Work out the finished part from the listing and answer in its coordinate system (mm). A direction names the side the tool comes from. Coordinates: 2 decimals unless noted, no trailing zeros. Write each loop counter-clockwise with the first axis right and the second up, starting at its lowest first coordinate (ties: lowest second). Pieces come first, ordered by that corner, then holes. Notation, with made-up numbers: M 73,9 L 129,9 A22 cw 129,19 Z; hole C -30,65 d1. An arc over 180 degrees is marked long. Answer as CSV lines item,"result". Start each with the question number.
(1) A cutting plane is placed at C-C on y = 19. Give the vertices of the cut face in (x, z), then the cut area to 3 significant figures.
(2) The mould has two halves that part along Y. Classify faces 4 (the cylindrical face through (33.538, 17.004, 6.014)), 5 (the flat face through (-17.75, 22, 6)), 6 (the cylindrical face through (-19.14, -26.1, 4.04)), 7 (the conical face through (30.577, -30.812, 0.125)): released by +Y, released by -Y, zero draft, split by the parting line, or undercut.
(3) Flat-ended cylindrical pins translate along their axes: P1, Ø4, axis at x = 30, y = 17.5, coming from the +Z side; P2, Ø5, axis at x = 24, z = 7, coming from the -Y side; P3, Ø1, axis at x = -24.5, z = 7.5, coming from the -Y side. Find the tip coordinate at first contact, or state that the pin passes through.
(4) Find the intervals of material crossed by L1, parallel to Y at x = 16, z = 6.45; L2, parallel to Y at x = -11.5, z = 5.25; L3, parallel to X at y = -24.5, z = 1.5, in increasing order. Write a range as [from, to].
(5) For faces 1 (the conical face through (29.334, -29.541, 1.347)), 2 (the flat face through (-32, -30, 6)), 3 (the flat face through (-19, 22, 4)), determine the directions among +Z, -Z, +X, -X, +Y, -Y from which every point of the face is accessible in a straight line to the end or side of a thin tool.
(6) A cutting plane is placed at B-B on y = -14. Give the vertices of the cut face in (x, z), then the cut area to 3 significant figures.
(7) A cutting plane is placed at A-A on x = 7.5. Give the vertices of the cut face in (y, z), then the cut area to 3 significant figures.
(8) A cutting plane is placed at D-D on x = 16. Give the vertices of the cut face in (y, z).
from build123d import *

# Parameters (mm, degrees)
PAD_DEPTH       = 9
POCKET_DEPTH    = 8
SKETCH002_W     = 37
SKETCH002_H     = 32
POCKET001_DEPTH = 1.001
POCKET002_DEPTH = 5
SKETCH004_W     = 45
SKETCH004_H     = 5
POCKET003_DEPTH = 74.001
SKETCH005_W     = 6.5
SKETCH005_H     = 8
PAD001_DEPTH    = 6
SKETCH006_R     = 2.25
POCKET004_DEPTH = 2
CHAMFER_SIZE    = 2
CHAMFER001_SIZE = 2
FILLET_R        = 3


with BuildPart() as part:
    # Sketch → Pad (new body)
    with BuildSketch(Plane.XY):
        with BuildLine():
            Line((-37, 23), (-37, -20))
            ThreePointArc((-37, -20), (-32.020815, -32.020815), (-20, -37))
            Line((-20, -37), (20.000003, -37))
            ThreePointArc((20.000003, -37), (32.020816, -32.020814), (37, -20))
            Line((37, -20), (37, 23))
            Line((-37, 23), (37, 23))
        make_face()
    extrude(amount=PAD_DEPTH)

    # Sketch001 (on Face8 of Pad) → Pocket (cut)
    with BuildSketch(Plane.XY.offset(9)):
        with BuildLine():
            Line((-35, 21), (-35, -20))
            ThreePointArc((-35, -20), (-30.606602, -30.606602), (-20, -35))
            Line((-20, -35), (20, -35))
            ThreePointArc((20, -35), (30.606602, -30.606602), (35, -20))
            Line((35, 21), (35, -20))
            Line((-35, 21), (35, 21))
        make_face()
    extrude(amount=-POCKET_DEPTH, mode=Mode.SUBTRACT)

    # Sketch002 (on Face15 of Pocket) → Pocket001 (cut, through all)
    with BuildSketch(Plane.XY.offset(1)):
        with Locations((3, 1)):
            Rectangle(SKETCH002_W, SKETCH002_H)
    extrude(amount=-POCKET001_DEPTH, mode=Mode.SUBTRACT)

    # Sketch003 (on Face2 of Pocket001) → Pocket002 (cut)
    with BuildSketch(Plane(origin=(0, 23, 0), x_dir=(-1, 0, 0), z_dir=(0, 1, 0))):
        Polygon((-35, 9), (35, 9), (35, 7), (24.25, 7), (24.25, 5), (23, 5), (23, 3), (19, 3), (19, 5), (17.75, 5), (17.75, 7), (-17.75, 7), (-17.75, 5), (-19, 5), (-19, 3), (-23, 3), (-23, 5), (-24.25, 5), (-24.25, 7), (-35, 7), align=None)
    extrude(amount=-POCKET002_DEPTH, mode=Mode.SUBTRACT)

    # Sketch004 → Pocket003 (cut, through all)
    with BuildSketch(Plane.YZ.offset(37)):
        with Locations((-7.5, 6.5)):
            Rectangle(SKETCH004_W, SKETCH004_H)
    extrude(amount=-POCKET003_DEPTH, mode=Mode.SUBTRACT)

    # Sketch005 (on Face43 of Pocket003) → Pad001 (join)
    with BuildSketch(Plane.XY.offset(1)):
        Polygon((-20, -19), (20, -19), (20, -27), (12, -27), (12, -21), (-12, -21), (-12, -27), (-20, -27), align=None)
        with Locations((-31.75, 18.9)):
            Rectangle(SKETCH005_W, SKETCH005_H)
        with Locations((31.75, 18.9)):
            Rectangle(SKETCH005_W, SKETCH005_H)
    extrude(amount=PAD001_DEPTH)

    # Sketch006 (on Face69 of Pad001) → Pocket004 (cut)
    with BuildSketch(Plane.XY.offset(7)):
        with Locations((-16, -23)):
            Circle(SKETCH006_R)
        with Locations((16, -23)):
            Circle(SKETCH006_R)
        with Locations((-32.5, 19)):
            Circle(SKETCH006_R)
        with Locations((32.5, 19)):
            Circle(SKETCH006_R)
    extrude(amount=-POCKET004_DEPTH, mode=Mode.SUBTRACT)

    # Chamfer
    chamfer_edges = [part.edges().sort_by_distance(p)[0] for p in [
        (-35, -2.55, 1),
    ]]
    chamfer(chamfer_edges, length=CHAMFER_SIZE)

    # Chamfer001
    chamfer001_edges = [part.edges().sort_by_distance(p)[0] for p in [
        (32.020816, -32.020814, 0),
    ]]
    chamfer(chamfer001_edges, length=CHAMFER001_SIZE)

    # Fillet
    fillet_edges = [part.edges().sort_by_distance(p)[0] for p in [
        (-28.5, 14.9, 4),
        (28.5, 14.9, 4),
        (20, -27, 4),
        (12, -27, 4),
        (-12, -27, 4),
        (-20, -27, 4),
        (-20, -19, 4),
        (20, -19, 4),
    ]]
    fillet(fillet_edges, radius=FILLET_R)


solid = part.part
Here are the results:
1,outline,"M -37,2 L -35,0 L 35,0 L 37,2 L 37,9 L 35,9 L 35,7 L 34.75,7 L 34.75,5 L 30.25,5 L 30.25,7 L 28.5,7 L 28.5,1 L -28.5,1 L -28.5,7 L -30.25,7 L -30.25,5 L -34.75,5 L -34.75,7 L -35,7 L -35,9 L -37,9 Z"
1,area,"162 mm^2"
2,face 4,"undercut"
2,face 5,"zero draft"
2,face 6,"undercut"
2,face 7,"released by -Y"
3,P1,"stops at z = 7"
3,P2,"stops at y = -36.93"
3,P3,"stops at y = -36.52"
4,L1,"y = [-37, -35], [-27, -25.25], [-20.75, -19], [21, 23]"
4,L2,"y = [-37, -35], [-21, -19], [21, 23]"
4,L3,"x = [-35.87, -32.73], [-19.96, -12.04], [12.04, 19.96], [32.73, 35.87]"
5,face 1,"+Z"
5,face 2,"+Z, +X, -X"
5,face 3,"+Z, +Y"
6,outline,"M -37,2 L -35,0 L -15.5,0 L -15.5,1 L -33,1 L -35,3 L -35,4 L -37,4 Z; M 21.5,0 L 35,0 L 37,2 L 37,4 L 35,4 L 35,3 L 33,1 L 21.5,1 Z"
6,area,"49.0 mm^2"
7,outline,"M -37,2 L -35,0 L -15,0 L -15,1 L -19,1 L -19,7 L -21,7 L -21,1 L -33,1 L -35,3 L -35,9 L -37,9 Z; M 17,0 L 23,0 L 23,7 L 21,7 L 21,1 L 17,1 Z"
7,area,"68.0 mm^2"
8,outline,"M -37,2 L -35,0 L -15,0 L -15,1 L -19,1 L -19,7 L -20.75,7 L -20.75,5 L -25.25,5 L -25.25,7 L -27,7 L -27,1 L -33,1 L -35,3 L -35,9 L -37,9 Z; M 17,0 L 23,0 L 23,7 L 21,7 L 21,1 L 17,1 Z"
